Design review of the part built by this model. Coordinates are the model's own, in mm. A direction names the side the tool comes from. Round coordinates to 2 decimals unless told otherwise and drop trailing zeros.
from build123d import *


with BuildPart() as part:
    # Sketch2 → Revolve1 (revolve)
    with BuildSketch(Plane.XY, mode=Mode.PRIVATE) as revolve1_sk:
        with BuildLine():
            Line((46.482, 0), (46.482, 91.948))
            Line((46.482, 91.948), (48.003200413, 91.948))
            ThreePointArc((48.003200413, 91.948), (38.343372168, 267.70619245), (10.118403547, 441.452))
            Line((10.118403547, 441.452), (10.118403547, 444.5))
            Line((10.118403547, 444.5), (12.573, 444.5))
            ThreePointArc((12.573, 444.5), (41.405749629, 267.738018442), (51.054, 88.9))
            Line((51.054, 88.9), (49.53, 88.9))
            Line((49.53, 88.9), (49.53, 0))
            Line((49.53, 0), (46.482, 0))
        make_face()
    revolve(revolve1_sk.sketch.rotate(Axis((0, 0, 0), (0, 1, 0)), 90), axis=Axis((0, 0, 0), (0, 1, 0)))


solid = part.part
1) The part is to be moulded in two halves that separate along Z. For faces 1 (the face through (-14.88, 43.83, -47.24)), 2 (the face through (-10.3, 444.5, 0.9)), 3 (the face through (45.377, 46.618, 10.076)), say which applies: released by +Z, released by -Z, zero draft, split by the parting line, or undercut.
Results:
face 1: split by the parting line
face 2: zero draft
face 3: undercut
2) To check wall thickness, follow line 1 along Z through (x, y) = (-24, 67); line 2 along Z through (x, y) = (2, 271.5); line 3 along X through (y, z) = (442.8, 0). State the ranges of each line that lie inside material, in increasing order.
Results:
line 1: z = -43.33 to -39.81, 39.81 to 43.33
line 2: z = -40.95 to -37.87, 37.87 to 40.95
line 3: x = -12.94 to -10.12, 10.12 to 12.94
3) Clearance check with flat-ended pins moving along their axes: P1, Ø2, axis at y = 191.5, z = -21.5, coming from the -X side; P2, Ø1.5, axis at y = 149.5, z = -19, coming from the -X side; P3, Ø2, axis at x = -18.5, y = 303.5, coming from the -Z side. State where each tip first meets the part, or that it passes through.
Results:
P1: stops at x = -43.28
P2: stops at x = -46.5
P3: stops at z = -32.78
4) For faces 4 (the face through (-14.9, 0, 44.3)), 5 (the face through (-39.34, 91.948, -25.11)), 6 (the face through (-42, 88.9, 27)), list the 3-axis set-ups (+Z, -Z, +X, -X, +Y, -Y) from which the entire face can be reached by the end or side of a thin tool; tool diameter is ignored.
Results:
face 4: +Z, -Z, +X, -X, -Y
face 5: none
face 6: -Y
